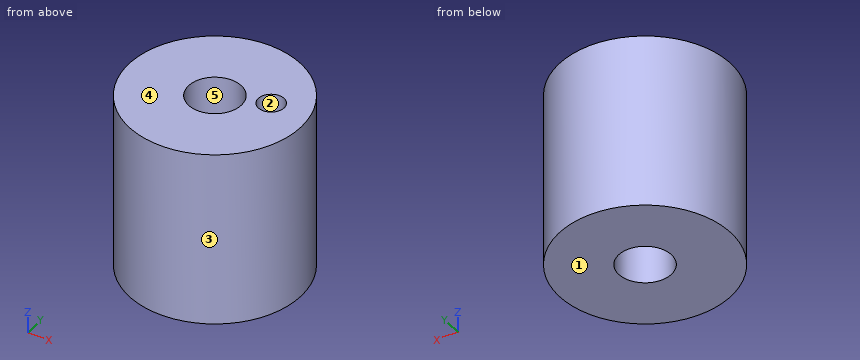
from build123d import *

# Parameters (mm, degrees)
F0_R     = 4.875
F1_DEPTH = 10
F2_R     = 1.5
F3_DEPTH = 10
F4_R     = 0.733358
F5_DEPTH = 3.3


with BuildPart() as f1:
    # F0 (on Top) → F1 (new body)
    with BuildSketch(Plane.XY):
        Circle(F0_R)
    extrude(amount=F1_DEPTH)

    # F2 (on face) → F3 (cut)
    with BuildSketch(Plane.XY.offset(10)):
        Circle(F2_R)
    extrude(amount=-F3_DEPTH, mode=Mode.SUBTRACT)

    # F4 (on face) → F5 (cut)
    with BuildSketch(Plane.XY.offset(10)):
        with Locations((2.626942, 0.882414)):
            Circle(F4_R)
    extrude(amount=-F5_DEPTH, mode=Mode.SUBTRACT)


solid = f1.part
Source: CAD feature listing. Evaluate the final solid. Frame: model axes, mm. Face numbers are marked on the shaded views. A direction names the side the tool comes from. Round coordinates to 2 decimals unless told otherwise and drop trailing zeros. Write each loop counter-clockwise with the first axis right and the second up, starting at its lowest first coordinate (ties: lowest second). Pieces come first, ordered by that corner, then holes. Notation, with made-up numbers: M -23.75,-12.5 L -8.75,-12.5 A23 ccw -8.75,6.5 Z; hole C 43.5,1.5 d2. An arc over 180 degrees is marked long. One line per item, written item: value. Start each with the question number.
Item 1: Section query D-D (y = 4). Return the cut outline in (x, z).
Item 2: Section query A-A (y = 0). Return the cut outline in (x, z) (3 decimals), plus the area to 3 significant figures.
Item 3: Ray query, L1, parallel to Y at x = 0, z = 7.5 (3 decimals); L2, parallel to X at y = -0.25, z = 5; L3, parallel to Y at x = 0.5, z = 7.5. Return the intervals inside material, ascending. Write a range as from..to.
Item 4: Mould query, pull axis X, two halves, no side actions, for the marked faces 3, 4 and 5. Classes: pulls with the +X half, pulls with the -X half, needs draft (parallel to the pull), parting line crosses it, or undercut.
Item 5: Pin query (flat end, axial travel): pin 1 (4 mm diameter, centred on y = -2.5, z = 3.5, fed in from -X); pin 2 (5 mm diameter, centred on x = -4, z = 4, fed in from -Y); pin 3 (1 mm diameter, centred on y = -2, z = 7, fed in from +X). Return the tip coordinate at first contact, or that it passes through.
Item 6: Section query C-C (z = 1). Return the cut outline in (x, y) (3 decimals), plus the area to 3 significant figures.
Item 7: Set-up query: the marked faces 1 and 2. Return all of +Z, -Z, +X, -X, +Y, -Y with unobstructed straight access to the full face (end or side cutting, diameter ignored); none if empty.
Result set:
1. outline: M -2.79,0 L 2.79,0 L 2.79,10 L -2.79,10 Z
2. outline: M -4.875,0 L -1.5,0 L -1.5,10 L -4.875,10 Z; M 1.5,0 L 4.875,0 L 4.875,10 L 1.5,10 Z
2. area: 67.5 mm²
3. L1: y = -4.875..-1.5, 1.5..4.875
3. L2: x = -4.87..-1.48, 1.48..4.87
3. L3: y = -4.85..-1.41, 1.41..4.85
4. face 3: parting line crosses it
4. face 4: needs draft
4. face 5: undercut
5. pin 1: stops at x = -4.85
5. pin 2: stops at y = -4.64
5. pin 3: stops at x = 4.64
6. outline: C 0,0 d9.75; hole C 0,0 d3
6. area: 67.6 mm²
7. face 1: -Z, +X, -X, +Y, -Y
7. face 2: +Z
